Model file for the job. Use its own axes, mm. Face numbers are marked on the shaded views. A direction names the side the tool comes from. Give positions to 0.01 mm unless a question says otherwise; leave off trailing zeros. Loops run counter-clockwise (first coordinate to the right, second up) from the corner with the lowest first, then second, coordinate; pieces in that order, holes last. Notation, with made-up numbers: M 75.25,17 L 95.25,17 A26 cw 95.25,54 Z; hole C 52,-3.5 d10. An arc over 180 degrees is marked long. Answer in a Markdown table with one row per item.
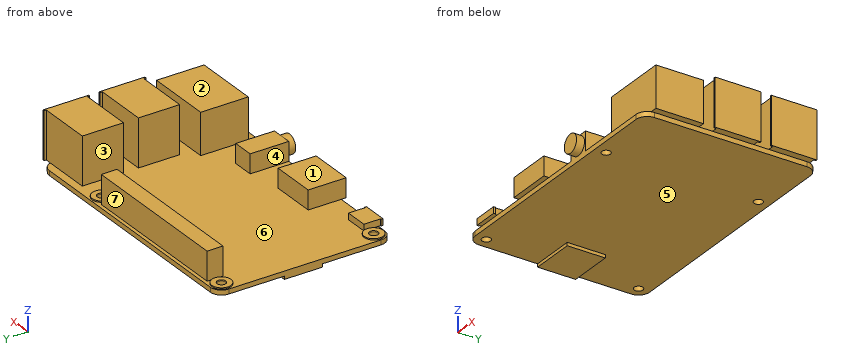
```python
from build123d import *

# Parameters (mm, degrees)
F1_DEPTH  = 0.75
F2_W      = 15.2527261972
F2_H      = 13
F3_DEPTH  = 15
F4_DEPTH  = 2
F5_W      = 50
F5_H      = 5
F6_DEPTH  = 9
F7_W      = 7.3
F7_H      = 4.5542112009
F7_W_2    = 14.2
F7_H_2    = 10.4107348667
F7_W_3    = 6.8
F7_H_3    = 12.2
F7_H_4    = 1.5892651333
F8_DEPTH  = 6
F9_DEPTH  = 4
F10_W     = 14
F10_H     = 12
F11_DEPTH = 1
F12_R     = 2.9
F13_DEPTH = 2.5
F14_R     = 3
F14_R_2   = 1.375
F15_DEPTH = 0.4
F16_DEPTH = 25


with BuildPart() as f1:
    # F0 (on Top) → F1 (new body, symmetric)
    with BuildSketch(Plane.XY):
        with BuildLine():
            Line((96.8816299438, 73.7570084287), (20.8816299438, 73.7570084287))
            ThreePointArc((20.8816299438, 73.7570084287), (18.4067562097, 72.7318821628), (17.3816299438, 70.2570084287))
            Line((17.3816299438, 70.2570084287), (17.3816299438, 22.2570084287))
            ThreePointArc((17.3816299438, 22.2570084287), (18.4067562097, 19.7821346945), (20.8816299438, 18.7570084287))
            Line((20.8816299438, 18.7570084287), (96.8816299438, 18.7570084287))
            ThreePointArc((96.8816299438, 18.7570084287), (99.356503678, 19.7821346945), (100.3816299438, 22.2570084287))
            Line((100.3816299438, 22.2570084287), (100.3816299438, 70.2570084287))
            ThreePointArc((100.3816299438, 70.2570084287), (99.356503678, 72.7318821628), (96.8816299438, 73.7570084287))
        make_face()
    extrude(amount=F1_DEPTH, both=True)

    # F2 (on face) → F3 (join)
    with BuildSketch(Plane.XY.offset(0.75)):
        with BuildLine():
            Line((100.2344762848, 71.2612103079), (85.1289037466, 71.2612103079))
            Line((85.1289037466, 71.2612103079), (85.1289037466, 58.2612103079))
            Line((85.1289037466, 58.2612103079), (100.3816299438, 58.2612103079))
            Line((100.3816299438, 58.2612103079), (100.3816299438, 70.2570084287))
            ThreePointArc((100.3816299438, 70.2570084287), (100.3446461287, 70.7644716327), (100.2344762848, 71.2612103079))
        make_face()
        with BuildLine():
            Line((102.1289037466, 71.2612103079), (100.2344762848, 71.2612103079))
            ThreePointArc((100.2344762848, 71.2612103079), (100.3446461287, 70.7644716327), (100.3816299438, 70.2570084287))
            Line((100.3816299438, 70.2570084287), (100.3816299438, 58.2612103079))
            Line((100.3816299438, 58.2612103079), (102.1289037466, 58.2612103079))
            Line((102.1289037466, 58.2612103079), (102.1289037466, 57.5612103079))
            Line((102.1289037466, 57.5612103079), (102.6289037466, 57.5612103079))
            Line((102.6289037466, 57.5612103079), (102.6289037466, 71.9612103079))
            Line((102.6289037466, 71.9612103079), (102.1289037466, 71.9612103079))
            Line((102.1289037466, 71.9612103079), (102.1289037466, 71.2612103079))
        make_face()
        Polygon((102.1210900545, 53.5538156629), (100.3816299438, 53.5538156629), (100.3816299438, 40.5538156629), (102.1289037466, 40.5538156629), (102.1289037466, 39.8538156629), (102.6289037466, 39.8538156629), (102.6289037466, 54.2538156629), (102.1210900545, 54.2538156629), align=None)
        with Locations((92.7552668452, 47.0538156629)):
            Rectangle(F2_W, F2_H)
        with BuildLine():
            Line((100.3816299438, 22.2570084287), (100.3816299438, 36.2560376525))
            Line((100.3816299438, 36.2560376525), (85.1289037466, 36.2560376525))
            Line((85.1289037466, 36.2560376525), (81.6289037466, 36.2560376525))
            Line((81.6289037466, 36.2560376525), (81.6289037466, 21.2560376525))
            Line((81.6289037466, 21.2560376525), (85.1289037466, 21.2560376525))
            Line((85.1289037466, 21.2560376525), (100.2354423276, 21.2560376525))
            ThreePointArc((100.2354423276, 21.2560376525), (100.3448902101, 21.7512136793), (100.3816299438, 22.2570084287))
        make_face()
        with BuildLine():
            Line((102.4976894259, 36.2560376525), (100.3816299438, 36.2560376525))
            Line((100.3816299438, 36.2560376525), (100.3816299438, 22.2570084287))
            ThreePointArc((100.3816299438, 22.2570084287), (100.3448902101, 21.7512136793), (100.2354423276, 21.2560376525))
            Line((100.2354423276, 21.2560376525), (102.4976894259, 21.2560376525))
            Line((102.4976894259, 21.2560376525), (102.4976894259, 36.2560376525))
        make_face()
    extrude(amount=F3_DEPTH)

    # F4 (cut): a face of the model
    f4_faces = [f1.faces().sort_by_distance(p)[0] for p in [
        (92.0632965863, 28.7560376525, 15.75),
    ]]
    extrude(f4_faces, amount=-F4_DEPTH, mode=Mode.SUBTRACT)

    # F5 (on face) → F6 (join)
    with BuildSketch(Plane.XY.offset(0.75)):
        with Locations((49.090506424, 70.1389685273)):
            Rectangle(F5_W, F5_H)
    extrude(amount=F6_DEPTH)

    # F7 (on face) → F8 (join)
    with BuildSketch(Plane.XY.offset(0.75)):
        with Locations((27.5762250692, 21.0341140292)):
            Rectangle(F7_W, F7_H)
        Polygon((31.2262250692, 18.7570084287), (23.9262250692, 18.7570084287), (23.9262250692, 18.1112196296), (23.6262250692, 18.1112196296), (23.6262250692, 17.4612196296), (31.5262250692, 17.4612196296), (31.5262250692, 18.1112196296), (31.2262250692, 18.1112196296), align=None)
        with Locations((48.5707884192, 23.9623758621)):
            Rectangle(F7_W_2, F7_H_2)
        with Locations((69.6124156952, 24.8570084287)):
            Rectangle(F7_W_3, F7_H_3)
        with Locations((48.5707884192, 17.9623758621)):
            Rectangle(F7_W_2, F7_H_4)
    extrude(amount=F8_DEPTH)

    # F9 (cut): a face of the model
    f9_faces = [f1.faces().sort_by_distance(p)[0] for p in [
        (27.5762250692, 20.3626902179, 6.75),
    ]]
    extrude(f9_faces, amount=-F9_DEPTH, mode=Mode.SUBTRACT)

    # F10 (on face) → F11 (join)
    with BuildSketch(Plane(origin=(0, 0, -0.75), x_dir=(1, 0, 0), z_dir=(0, 0, -1))):
        with Locations((24.3816299438, -46.7570084287)):
            Rectangle(F10_W, F10_H)
    extrude(amount=F11_DEPTH)

    # F12 (on face) → F13 (join)
    with BuildSketch(Plane.XZ.offset(-18.7570084287)):
        with Locations((69.6124156952, 3.75)):
            Circle(F12_R)
    extrude(amount=F13_DEPTH)

    # F14 (on face) → F15 (join)
    with BuildSketch(Plane.XY.offset(0.75)):
        with Locations((77.4679929018, 70.2570084287)):
            Circle(F14_R)
        with Locations((77.4679929018, 70.2570084287)):
            Circle(F14_R_2, mode=Mode.SUBTRACT)
        with Locations((20.8816299438, 70.2570084287)):
            Circle(F14_R)
        with Locations((20.8816299438, 70.2570084287)):
            Circle(F14_R_2, mode=Mode.SUBTRACT)
        with Locations((20.8816299438, 22.2570084287)):
            Circle(F14_R)
        with Locations((20.8816299438, 22.2570084287)):
            Circle(F14_R_2, mode=Mode.SUBTRACT)
        with Locations((77.4679929018, 22.2570084287)):
            Circle(F14_R)
        with Locations((77.4679929018, 22.2570084287)):
            Circle(F14_R_2, mode=Mode.SUBTRACT)
    extrude(amount=F15_DEPTH)

    # F16 (cut): faces of the model
    f16_faces = [f1.faces().sort_by_distance(p)[0] for p in [
        (77.4679929018, 70.2570084287, 0.75),
        (77.4679929018, 22.2570084287, 0.75),
        (20.8816299438, 22.2570084287, 0.75),
        (20.8816299438, 70.2570084287, 0.75),
    ]]
    extrude(f16_faces, amount=-F16_DEPTH, mode=Mode.SUBTRACT)


solid = f1.part
```
Q1. Probe probe 1 along Y at (x, z) = (89, 1); probe 2 along Y at (x, z) = (49.5, 2.25); probe 3 along Z at (x, y) = (73.5, 33.5). List the from-to ranges inside material, lowest first.
Reported:
| item | result |
|---|---|
| probe 1 | 21.26 to 36.26, 40.55 to 53.55, 58.26 to 71.26 |
| probe 2 | 17.17 to 29.17, 67.64 to 72.64 |
| probe 3 | -0.75 to 0.75 |
Q2. Saw through at B-B (x = 92.5). Give the cut face in (y, z), and give its area (4 significant figures).
Reported:
| item | result |
|---|---|
| outline | M 18.76,-0.75 L 73.76,-0.75 L 73.76,0.75 L 71.26,0.75 L 71.26,15.75 L 58.26,15.75 L 58.26,0.75 L 53.55,0.75 L 53.55,15.75 L 40.55,15.75 L 40.55,0.75 L 36.26,0.75 L 36.26,13.75 L 21.26,13.75 L 21.26,0.75 L 18.76,0.75 Z |
| area | 667.5 mm² |
Q3. Saw through at D-D (y = 60). Give the cut face in (x, z).
Reported:
| item | result |
|---|---|
| outline | M 17.38,-0.75 L 100.38,-0.75 L 100.38,0.75 L 102.63,0.75 L 102.63,15.75 L 85.13,15.75 L 85.13,0.75 L 17.38,0.75 Z |
Q4. Drop flat-ended pins along their axis: pin 1 (1.6 mm diameter, centred on y = 38.5, z = 0, fed in from +X); pin 2 (1.1 mm diameter, centred on x = 102, y = 29.5, fed in from -Z); pin 3 (6.5 mm diameter, centred on x = 77, y = 23.5, fed in from +Z). Give the stop position or say it passes through.
Reported:
| item | result |
|---|---|
| pin 1 | x = 100.38 |
| pin 2 | z = 0.75 |
| pin 3 | z = 1.15 |
Q5. 3-axis set-ups, long thin cutter, end or side, ignore diameter. For the marked faces 1, 2, 3 and 4: which of +Z, -Z, +X, -X, +Y, -Y reach the whole face in a straight line?
Reported:
| item | result |
|---|---|
| face 1 | +Z, -X, -Y |
| face 2 | +Z, +X, -X, -Y |
| face 3 | +Z, +Y |
| face 4 | +Z, -Y |
Q6. Mould opens along Y. For the marked faces 5, 6 and 7 say: released by +Y, released by -Y, zero draft, split by the parting line, or undercut.
Reported:
| item | result |
|---|---|
| face 5 | zero draft |
| face 6 | undercut |
| face 7 | released by +Y |
Q7. Saw through at A-A (y = 34). Give the cut face in (x, z), and give its area (3 significant figures).
Reported:
| item | result |
|---|---|
| outline | M 17.38,-0.75 L 100.38,-0.75 L 100.38,0.75 L 102.5,0.75 L 102.5,13.75 L 81.63,13.75 L 81.63,0.75 L 17.38,0.75 Z |
| area | 396 mm² |
Q8. Saw through at C-C (z = 3.75). Give the number of separate pieces and of enclosed holes in the cut face, and give its area (3 significant figures).
Reported:
| item | result |
|---|---|
| separate pieces | 6 |
| enclosed holes | 0 |
| area | 1,290 mm² |
